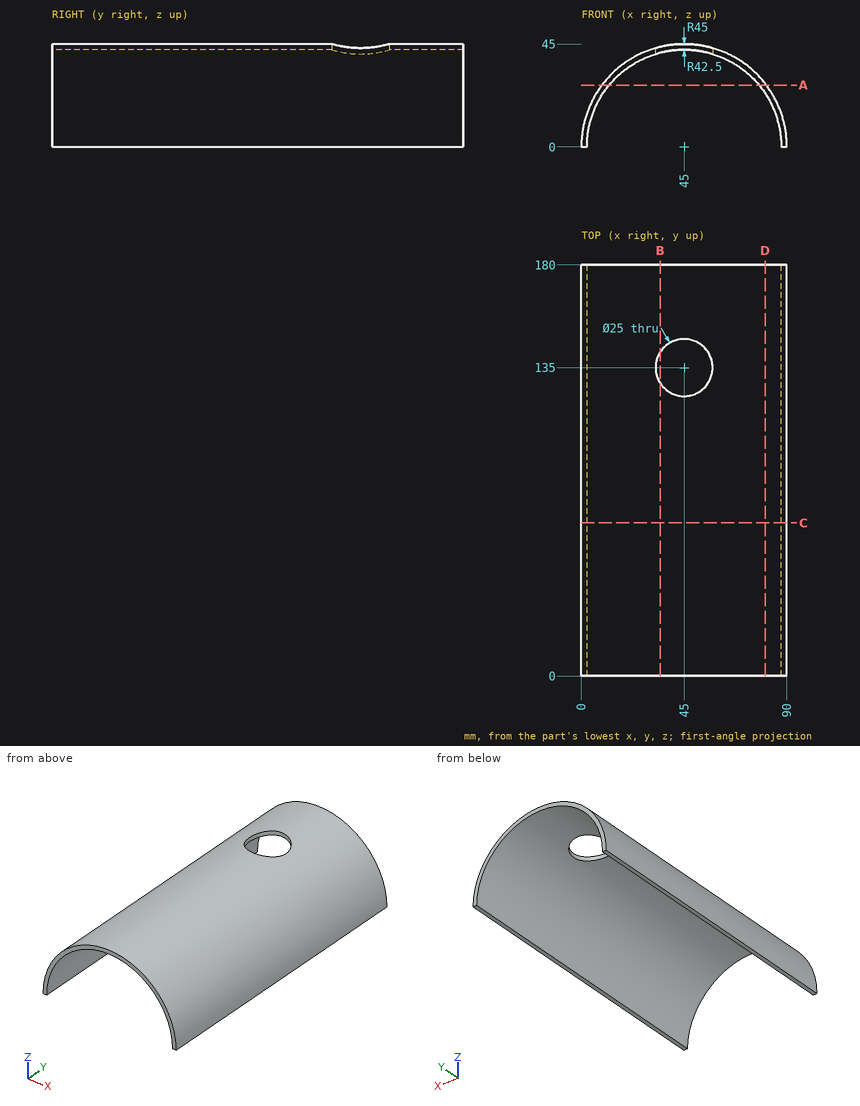
Design review of the part shown in the three views and the two pictorial views. Dimensions are in mm from the part's minimum x, y and z. Give positions to 0.01 mm unless a question says otherwise; leave off trailing zeros. Write each loop counter-clockwise with the first axis right and the second up, starting at its lowest first coordinate (ties: lowest second). Pieces come first, ordered by that corner, then holes. Notation, with made-up numbers: (25.5, -27.5) - (30.5, -27.5) arc R3 ccw to (30.5, -22.5) - close; hole circle Ø2 at (58, -2). An arc over 180 degrees is marked (long way). Return JSON: item names as keys, results as strings. Group by question number.
(1) We need section D-D, the plane x = 80.5. Give the boundary of the cut face in (y, z), then the cut area to 3 significant figures.
(2) We need section B-B, the plane x = 34.5. Give the boundary of the cut face in (y, z), then the cut area to 3 significant figures.
(3) Insertion check: pin 1 (6 mm diameter, centred on x = 66.5, y = 147, fed in from -Z); pin 2 (8 mm diameter, centred on x = 75, y = 95.5, fed in from +Z); pin 3 (4 mm diameter, centred on x = 28, y = 26.5, fed in from +Z); pin 4 (12 mm diameter, centred on x = 51, z = 35.5, fed in from +Y). Each pin has a flat end and moves straight along its axis. Give the tip position at first contact, or say it passes through.
(4) To check wall thickness, follow probe 1 along Y at (x, z) = (45, 43.2); probe 2 along Z at (x, y) = (46.5, 164) (3 decimals); probe 3 along X at (y, z) = (133, 41.5). State the ranges of each line that lie inside material, in increasing order.
(5) We need section C-C, the plane y = 67. Give the boundary of the cut face in (x, z).
(6) We need section A-A, the plane z = 27. Give the boundary of the cut face in (x, y), then the cut area to 3 significant figures.
Reported:
{
 "1": {"outline": "(0, 23.37) - (180, 23.37) - (180, 27.65) - (0, 27.65) - close", "area": "772 mm2"},
 "2": {"outline": "(0, 41.18) - (128.22, 41.18) - (128.22, 43.76) - (0, 43.76) - close; (141.78, 41.18) - (180, 41.18) - (180, 43.76) - (141.78, 43.76) - close", "area": "429 mm2"},
 "3": {"pin 1": "stops at z = 34.73", "pin 2": "stops at z = 36.73", "pin 3": "stops at z = 42.43", "pin 4": "passes through"},
 "4": {"probe 1": "y = 0 to 122.5, 147.5 to 180", "probe 2": "z = 42.474 to 44.975", "probe 3": "x = 27.6 to 32.66, 57.34 to 62.4"},
 "5": {"outline": "(0, 0) - (2.5, 0) arc R42.5 cw to (87.5, 0) - (90, 0) arc R45 ccw to start"},
 "6": {"outline": "(9, 0) - (12.18, 0) - (12.18, 180) - (9, 180) - close; (77.82, 0) - (81, 0) - (81, 180) - (77.82, 180) - close", "area": "1,140 mm2"}
}
